Check sheet for the drawn part. Datum: minimum x, y, z corner. Units: mm. Give positions to 0.01 mm unless a question says otherwise; leave off trailing zeros. Write each loop counter-clockwise with the first axis right and the second up, starting at its lowest first coordinate (ties: lowest second). Pieces come first, ordered by that corner, then holes.
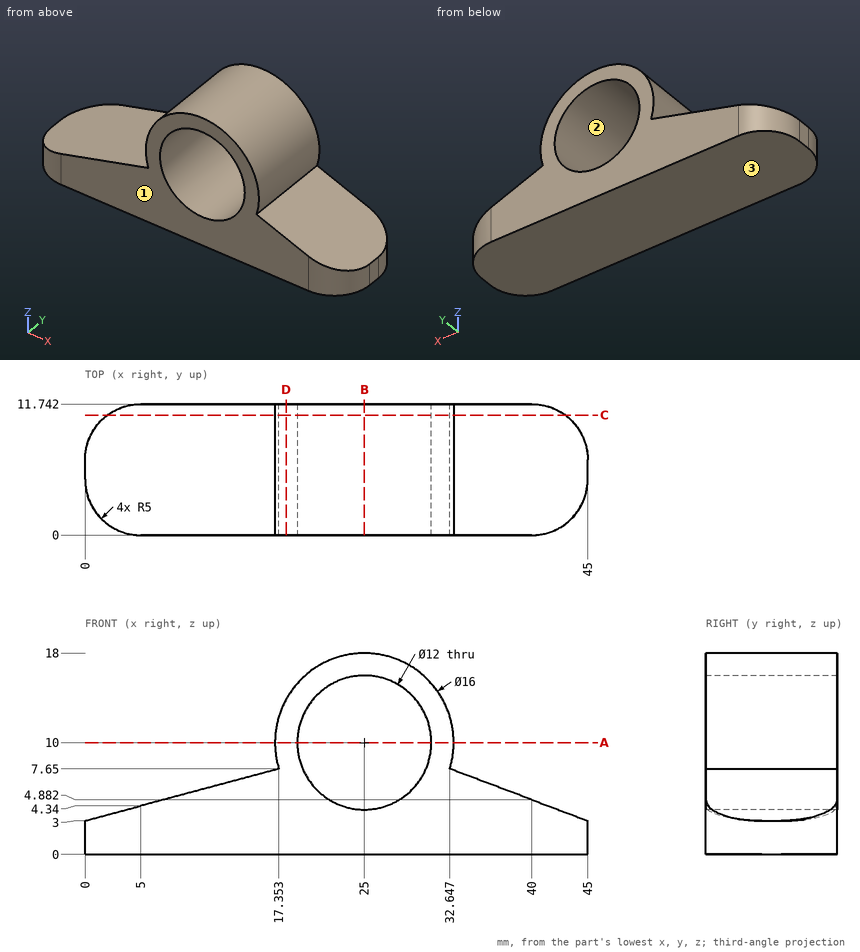
1) Scan lines: L1, parallel to X at y = 10.75, z = 10.25 (1 decimal); L2, parallel to Z at x = 25, y = 5.75; L3, parallel to Z at x = 29.5, y = 3 (1 decimal). Record each from-to range of solid material in increasing order.
2) Sectioned sample at B-B on x = 25. Record the boundary of the cut face in (y, z).
3) Draft check along Z on the marked faces 1, 2 and 3. Enter one of: +Z half, -Z half, draft (parallel to the pull), parting line (faces both ways), or undercut.
4) Sectioned sample at C-C on y = 10.75. Record the boundary of the cut face in (x, z).
5) Sectioned sample at A-A on z = 10. Record the boundary of the cut face in (x, y).
6) Gauge pin test, flat ends, axial feed: pin 1 (3 mm diameter, centred on x = 5, y = 4.5, fed in from -Z); pin 2 (1.5 mm diameter, centred on x = 23, y = 3.5, fed in from +Z); pin 3 (6 mm diameter, centred on y = 7.5, z = 14.5, fed in from +X). Record the tip position at first contact, or that the pin passes through.
7) Sectioned sample at D-D on x = 18. Record the boundary of the cut face in (y, z).
Answers below:
1. L1: x = 17 to 19, 31 to 33
1. L2: z = 0 to 4, 16 to 18
1. L3: z = 0 to 6, 14 to 16.6
2. outline: (0, 0) - (11.74, 0) - (11.74, 4) - (0, 4) - close; (0, 16) - (11.74, 16) - (11.74, 18) - (0, 18) - close
3. face 1: draft
3. face 2: undercut
3. face 3: -Z half
4. outline: (2.01, 0) - (42.99, 0) - (42.99, 3.76) - (32.65, 7.65) arc R8 ccw (long way) to (17.35, 7.65) - (2.01, 3.54) - close; hole circle Ø12 at (25, 10)
5. outline: (17, 0) - (19, 0) - (19, 11.74) - (17, 11.74) - close; (31, 0) - (33, 0) - (33, 11.74) - (31, 11.74) - close
6. pin 1: stops at z = 0
6. pin 2: stops at z = 17.9
6. pin 3: stops at x = 32.86
7. outline: (0, 0) - (11.74, 0) - (11.74, 13.87) - (0, 13.87) - close
